Model file for the job. Use its own axes, mm. A direction names the side the tool comes from. Round coordinates to 2 decimals unless told otherwise and drop trailing zeros. Loops run counter-clockwise (first coordinate to the right, second up) from the corner with the lowest first, then second, coordinate; pieces in that order, holes last.
from build123d import *

# Parameters (mm, degrees)
SKETCH1_R           = 34
BOSS_EXTRUDE1_DEPTH = 4
HOLE1_D             = 3
HOLE1_DEPTH         = 5
HOLE1_CBORE_D       = 6
HOLE1_CBORE_DEPTH   = 1.5
SKETCH2_R           = 17
CUT_EXTRUDE1_DEPTH  = 5


with BuildPart() as part:
    # Sketch1 → Boss-Extrude1 (new body)
    with BuildSketch(Plane(origin=(0, 0, 0), x_dir=(1, 0, 0), z_dir=(0, 1, 0))):
        Circle(SKETCH1_R)
    extrude(amount=BOSS_EXTRUDE1_DEPTH)

    # Hole1
    with Locations(Plane(origin=(0, 4, -25), x_dir=(0, 0, 1), z_dir=(0, 1, 0))):
        with Locations((0, 0), (12.5, 21.650635095), (37.5, 21.650635095), (50, 0), (37.5, -21.650635095), (12.5, -21.650635095)):
            CounterBoreHole(HOLE1_D / 2, HOLE1_CBORE_D / 2, HOLE1_CBORE_DEPTH, depth=HOLE1_DEPTH)

    # Sketch2 → Cut-Extrude1 (cut)
    with BuildSketch(Plane(origin=(0, 4, 0), x_dir=(1, 0, 0), z_dir=(0, 1, 0))):
        Circle(SKETCH2_R)
    extrude(amount=-CUT_EXTRUDE1_DEPTH, mode=Mode.SUBTRACT)


solid = part.part
Q1. Tool access for faces 1 (the face through (0, 3, 22)), 2 (the face through (0.07, 1.23, -23.5)): list every direction of +Z, -Z, +X, -X, +Y, -Y with a clear straight run to the whole face (end or side of a thin tool).
Q2. Slice it at C-C on y = 0.6. Give the cut face in (x, z), plus the area to 3 significant figures.
Q3. Flat gauge pins, fed straight in: P1, Ø5, axis at x = 21.65, z = 12.5, coming from the -Y side; P2, Ø5, axis at x = -21.65, z = 12.5, coming from the +Y side; P3, Ø1, axis at x = 21, y = 3, coming from the -Z side. Where does each tip first touch, or does it go through?
Q4. Probe line 1 (X direction, y = 3.05, z = 12.5); line 2 (Z direction, x = -1, y = 3.05); line 3 (X direction, y = 1.1, z = -5). List the from-to ranges inside material, lowest first.
Q5. Slice it at D-D on z = -12.5. Give the cut face in (x, y), plus the area to 3 significant figures.
Q6. Slice it at B-B on x = -14. Give the cut face in (y, z), plus the area to 3 significant figures.
Q7. Slice it at A-A on z = 0. Give the cut face in (x, y), plus the area to 3 significant figures.
Reply:
1. face 1: +Y
1. face 2: +Y, -Y
2. outline: circle Ø68 at (0, 0); hole circle Ø3 at (-21.65, -12.5); hole circle Ø3 at (-21.65, 12.5); hole circle Ø34 at (0, 0); hole circle Ø3 at (0, -25); hole circle Ø3 at (0, 25); hole circle Ø3 at (21.65, -12.5); hole circle Ø3 at (21.65, 12.5)
2. area: 2,680 mm2
3. P1: stops at y = 0
3. P2: stops at y = 2.5
3. P3: stops at z = -27.12
4. line 1: x = -31.62 to -24.65, -18.65 to -11.52, 11.52 to 18.65, 24.65 to 31.62
4. line 2: z = -33.99 to -27.83, -22.17 to -16.97, 16.97 to 22.17, 27.83 to 33.99
4. line 3: x = -33.63 to -16.25, 16.25 to 33.63
5. outline: (-31.62, 0) - (-23.15, 0) - (-23.15, 2.5) - (-24.65, 2.5) - (-24.65, 4) - (-31.62, 4) - close; (-20.15, 0) - (-11.52, 0) - (-11.52, 4) - (-18.65, 4) - (-18.65, 2.5) - (-20.15, 2.5) - close; (11.52, 0) - (20.15, 0) - (20.15, 2.5) - (18.65, 2.5) - (18.65, 4) - (11.52, 4) - close; (23.15, 0) - (31.62, 0) - (31.62, 4) - (24.65, 4) - (24.65, 2.5) - (23.15, 2.5) - close
5. area: 128 mm2
6. outline: (0, -30.98) - (4, -30.98) - (4, -9.64) - (0, -9.64) - close; (0, 9.64) - (4, 9.64) - (4, 30.98) - (0, 30.98) - close
6. area: 171 mm2
7. outline: (-34, 0) - (-17, 0) - (-17, 4) - (-34, 4) - close; (17, 0) - (34, 0) - (34, 4) - (17, 4) - close
7. area: 136 mm2
